Input: part model. Units: mm. Frame: model coordinates. Coordinates: 2 decimals unless noted, no trailing zeros. Order: outer loops, then holes, each group sorted by start corner. A loop starts at its lowest first (then second) coordinate and runs counter-clockwise, first axis right, second up. Notation, with made-up numbers: (63.5, 23.25) - (80.5, 23.25) arc R23 ccw to (80.5, 52.25) - close; hole circle Ø5 at (80, 62). An arc over 180 degrees is marked (long way). Use a Markdown table: item, result. Add a question column.
from build123d import *

# Parameters (mm, degrees)
BOSS_EXTRUDE1_DEPTH = 10
CUT_EXTRUDE1_DEPTH  = 10
SKETCH3_R           = 17.5
CUT_EXTRUDE2_DEPTH  = 10


with BuildPart() as part:
    # Sketch1 → Boss-Extrude1 (new body)
    with BuildSketch(Plane.XY):
        Polygon((-162.542296849, -28.60707156), (-158.542296849, -28.60707156), (-158.542296849, -64.60707156), (-153.542296849, -69.60707156), (-87.954361389, -69.60707156), (-12.936677956, 5.002214078), (39.495227245, 120.053529566), (34.542546963, 133.300074701), (1.783941212, 148.229031436), (3.442714182, 151.86887652), (-80.294668817, 151.86887652), align=None)
    extrude(amount=BOSS_EXTRUDE1_DEPTH)

    # Sketch2 → Cut-Extrude1 (cut)
    with BuildSketch(Plane.XY.offset(10)):
        Polygon((1.783941212, 148.229031436), (-77.953441788, 148.229031436), (-158.542296849, -28.60707156), (-177.628261738, -46.12321945), (-258.764859666, -56.78409298), (-118.247869319, 215.351823208), (19.357832203, 157.605676218), align=None)
    extrude(amount=-CUT_EXTRUDE1_DEPTH, mode=Mode.SUBTRACT)

    # Sketch3 → Cut-Extrude2 (cut)
    with BuildSketch(Plane(origin=(0, 0, 0), x_dir=(-1, 0, 0), z_dir=(0, 0, -1))):
        with Locations((37.542296849, 90.39292844)):
            Circle(SKETCH3_R)
    extrude(amount=-CUT_EXTRUDE2_DEPTH, mode=Mode.SUBTRACT)


solid = part.part
1) Cut plane C-C (x = 15.5). Return the cut outline in (y, z).
2) Pull-direction query (X, two-part tool) for faces 1 (the cylindrical face through (-45.62, 74.87, 4.93)), 2 (the flat face through (18.39, 140.66, 4.93)), 3 (the flat face through (-156.08, -67.07, 4.93)); classes: pulls with the +X half, pulls with the -X half, needs draft (parallel to the pull), parting line crosses it, or undercut.
3) Cut plane B-B (z = 7). Return the cut outline in (x, y).
4) Cut plane D-D (y = 2). Return the cut outline in (x, z).
5) Contact query for flat-ended pins moving along their axis: P1, Ø6, axis at x = -7.5, z = 5.5, coming from the -Y side; P2, Ø4, axis at y = -21.5, z = 7.5, coming from the +X side; P3, Ø4, axis at y = 1.5, z = 8.5, coming from the -X side. Output: stop coordinate, or through.
6) Material intervals for L1, parallel to Y at x = -51, z = 4.75; L2, parallel to X at y = 75, z = 7; L3, parallel to Y at x = -18, z = 9.25, sorted ascending.
7) Cut plane A-A (y = 103). Return the cut outline in (x, z).
Computed:
| question | item | result |
|---|---|---|
| 1 | outline | (67.4, 0) - (141.98, 0) - (141.98, 10) - (67.4, 10) - close |
| 2 | face 1 | undercut |
| 2 | face 2 | pulls with the +X half |
| 2 | face 3 | pulls with the -X half |
| 3 | outline | (-158.54, -64.61) - (-153.54, -69.61) - (-87.95, -69.61) - (-12.94, 5) - (39.5, 120.05) - (34.54, 133.3) - (1.78, 148.23) - (-77.95, 148.23) - (-158.54, -28.61) - close; hole circle Ø35 at (-37.54, 90.39) |
| 4 | outline | (-144.59, 0) - (-15.96, 0) - (-15.96, 10) - (-144.59, 10) - close |
| 5 | P1 | stops at y = 10.35 |
| 5 | P2 | stops at x = -37.57 |
| 5 | P3 | stops at x = -145.73 |
| 6 | L1 | y = -32.85 to 79.21, 101.58 to 148.23 |
| 6 | L2 | x = -111.33 to -45.87, -29.22 to 18.96 |
| 6 | L3 | y = -0.03 to 148.23 |
| 7 | outline | (-98.57, 0) - (-49.68, 0) - (-49.68, 10) - (-98.57, 10) - close; (-25.41, 0) - (31.72, 0) - (31.72, 10) - (-25.41, 10) - close |
